For this review, take the finished solid that the model builds, in its own axes (mm). Face numbers are marked on the shaded views. A direction names the side the tool comes from. Round coordinates to 2 decimals unless told otherwise and drop trailing zeros. Order: outer loops, then holes, each group sorted by start corner. A loop starts at its lowest first (then second) coordinate and runs counter-clockwise, first axis right, second up. Notation, with made-up numbers: M 47.5,49.5 L 90.5,49.5 A13 ccw 90.5,69.5 Z; hole C 38.25,78.25 d9. An arc over 180 degrees is marked long. Use a Markdown table: item, result.
from build123d import *

# Parameters (mm, degrees)
BOSS_EXTRUDE1_DEPTH      = 25.8
BOSS_EXTRUDE1_DEPTH_BACK = 25.8
CUT_EXTRUDE2_DEPTH       = 105.5
FILLET3_R                = 2
FILLET2_R                = 5
SKETCH4_R                = 2.3
BOSS_EXTRUDE2_DEPTH      = 9
SKETCH8_W                = 9.403990972
SKETCH8_H                = 11.260041821
SKETCH8_W_2              = 16.148154032
SKETCH8_H_2              = 11.415373045
CUT_EXTRUDE5_DEPTH       = 10
CUT_EXTRUDE6_DEPTH       = 56
CUT_EXTRUDE7_DEPTH       = 56
SKETCH11_W               = 6
SKETCH11_H               = 6
BOSS_EXTRUDE3_DEPTH      = 4
SKETCH12_R               = 1.25
CUT_EXTRUDE8_DEPTH       = 7
SKETCH13_W               = 5
SKETCH13_H               = 2.5
CUT_EXTRUDE9_DEPTH       = 4.5


with BuildPart() as part:
    # Sketch1 → Boss-Extrude1 (new, two sides: drawn at the far end of the back side and taken through both)
    with BuildSketch(Plane(origin=(0, 0, 0), x_dir=(0, 0, -1), z_dir=(1, 0, 0)).offset(-BOSS_EXTRUDE1_DEPTH_BACK)):
        Polygon((-45.5, 0), (-45.5, 21.5), (45.5, 21.5), (45.5, 0), (47.5, 0), (47.5, 23.5), (-47.5, 23.5), (-47.5, 0), align=None)
    extrude(amount=BOSS_EXTRUDE1_DEPTH + BOSS_EXTRUDE1_DEPTH_BACK)

    # Sketch3 → Cut-Extrude2 (cut)
    with BuildSketch(Plane(origin=(0, 0, -47.5), x_dir=(-1, 0, 0), z_dir=(0, 0, -1))):
        Polygon((-25.8, 21.5), (-24.65, 0), (-25.8, 0), align=None)
        Polygon((25.8, 21.5), (24.65, 0), (25.8, 0), align=None)
    extrude(amount=-CUT_EXTRUDE2_DEPTH, mode=Mode.SUBTRACT)

    # Fillet3
    fillet3_edges = [part.edges().sort_by_distance(p)[0] for p in [
        (24.65, 0, -46.5),
        (24.65, 0, 46.5),
        (-24.65, 0, -46.5),
        (-24.65, 0, 46.5),
    ]]
    fillet(fillet3_edges, radius=FILLET3_R)

    # Fillet2
    fillet2_edges = [part.edges().sort_by_distance(p)[0] for p in [
        (0, 21.5, 45.5),
        (0, 23.5, 47.5),
        (0, 23.5, -47.5),
        (0, 21.5, -45.5),
    ]]
    fillet(fillet2_edges, radius=FILLET2_R)

    # Sketch4 → Boss-Extrude2 (add)
    with BuildSketch(Plane.XZ.offset(-21.5)):
        with Locations(Location((-18.5, -26, 0), (0, 0, 270))):
            Circle(SKETCH4_R)
        with Locations(Location((18.5, -26, 0), (0, 0, 270))):
            Circle(SKETCH4_R)
        with Locations(Location((-18.5, 26, 0), (0, 0, 270))):
            Circle(SKETCH4_R)
        with Locations(Location((18.5, 26, 0), (0, 0, 270))):
            Circle(SKETCH4_R)
    extrude(amount=BOSS_EXTRUDE2_DEPTH)

    # Sketch8 → Cut-Extrude5 (cut)
    with BuildSketch(Plane.XY.offset(47.5)):
        with Locations((-10.345619811, 9.988318774)):
            Rectangle(SKETCH8_W, SKETCH8_H)
        with Locations((9.712305605, 7.570757784)):
            Rectangle(SKETCH8_W_2, SKETCH8_H_2)
    extrude(amount=-CUT_EXTRUDE5_DEPTH, mode=Mode.SUBTRACT)

    # Sketch9 → Cut-Extrude6 (cut)
    with BuildSketch(Plane(origin=(25.8, 0, 0), x_dir=(0, 0, -1), z_dir=(1, 0, 0))):
        with BuildLine():
            Line((-22.5, 23.5), (-22.5, 22.498632165))
            Line((-22.5, 22.498632165), (42.604598318, 22.498632165))
            ThreePointArc((42.604598318, 22.498632165), (45.365169565, 21.291201061), (46.5, 18.5))
            Line((46.5, 18.5), (46.5, 1.893175959))
            Line((46.5, 1.893175959), (47.5, 1.893175959))
            Line((47.5, 1.893175959), (47.5, 18.5))
            ThreePointArc((47.5, 18.5), (46.035533906, 22.035533906), (42.5, 23.5))
            Line((42.5, 23.5), (-22.5, 23.5))
        make_face()
    extrude(amount=-CUT_EXTRUDE6_DEPTH, mode=Mode.SUBTRACT)

    # Sketch10 → Cut-Extrude7 (cut)
    with BuildSketch(Plane(origin=(0, 22.498632165, 0), x_dir=(1, 0, 0), z_dir=(0, 1, 0))):
        Polygon((-22.8, -22.5), (-22.8, 21.604598318), (-12.8, 21.604598318), (-12.8, 29.604598318), (-22.8, 29.604598318), (-22.8, 38.604598318), (23.045882962, 38.604598318), (23.045882962, 29.604598318), (13.045882962, 29.604598318), (13.045882962, 21.604598318), (23.045882962, 21.604598318), (23.045882962, -22.5), align=None)
    extrude(amount=-CUT_EXTRUDE7_DEPTH, mode=Mode.SUBTRACT)

    # Sketch11 → Boss-Extrude3 (add)
    with BuildSketch(Plane(origin=(0, 0, -46.5), x_dir=(-1, 0, 0), z_dir=(0, 0, -1))):
        with Locations((-14.195398892, 10.196587979)):
            Rectangle(SKETCH11_W, SKETCH11_H)
        with Locations((14.195398892, 10.196587979)):
            Rectangle(SKETCH11_W, SKETCH11_H)
    extrude(amount=-BOSS_EXTRUDE3_DEPTH)

    # Sketch12 → Cut-Extrude8 (cut)
    with BuildSketch(Plane(origin=(0, 0, -46.5), x_dir=(-1, 0, 0), z_dir=(0, 0, -1))):
        with Locations((14.195398892, 10.196587979)):
            Circle(SKETCH12_R)
        with Locations((-14.195398892, 10.196587979)):
            Circle(SKETCH12_R)
    extrude(amount=-CUT_EXTRUDE8_DEPTH, mode=Mode.SUBTRACT)

    # Sketch13 → Cut-Extrude9 (cut)
    with BuildSketch(Plane(origin=(0, 13.196587979, 0), x_dir=(1, 0, 0), z_dir=(0, 1, 0))):
        with Locations((14.195398892, 44.25)):
            Rectangle(SKETCH13_W, SKETCH13_H)
        with Locations((-14.195398892, 44.25)):
            Rectangle(SKETCH13_W, SKETCH13_H)
    extrude(amount=-CUT_EXTRUDE9_DEPTH, mode=Mode.SUBTRACT)


solid = part.part
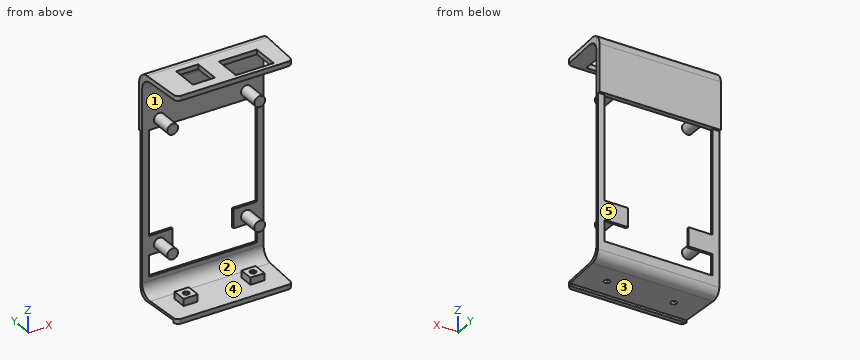
Q1. Draft analysis for pull direction X (two halves, no side actions). For the marked faces 4 and 5, state which applies: pulls with the +X half, pulls with the -X half, needs draft (parallel to the pull), parting line crosses it, or undercut.
Determined:
| item | result |
|---|---|
| face 4 | undercut |
| face 5 | needs draft |
Q2. Add section A-A (x = 0). Write out the cut boundary in (y, z).
Determined:
| item | result |
|---|---|
| outline | M 0,-47.5 L 1.89,-47.5 L 1.89,-46.5 L 18.5,-46.5 A4 ccw 22.5,-42.6 L 22.5,-38.6 L 21.5,-38.6 L 21.5,-40.5 A5 cw 16.5,-45.5 L 0,-45.5 Z; M 0,45.5 L 16.5,45.5 A5 cw 21.5,40.5 L 21.5,22.5 L 23.5,22.5 L 23.5,42.5 A5 ccw 18.5,47.5 L 0,47.5 Z |
Q3. Add section B-B (x = 9.5). Write out the cut boundary in (y, z).
Determined:
| item | result |
|---|---|
| outline | M 0,-47.5 L 1.89,-47.5 L 1.89,-46.5 L 18.5,-46.5 A4 ccw 22.5,-42.6 L 22.5,-38.6 L 21.5,-38.6 L 21.5,-40.5 A5 cw 16.5,-45.5 L 0,-45.5 Z; M 0,45.5 L 1.86,45.5 L 1.86,47.5 L 0,47.5 Z; M 13.28,45.5 L 16.5,45.5 A5 cw 21.5,40.5 L 21.5,22.5 L 23.5,22.5 L 23.5,42.5 A5 ccw 18.5,47.5 L 13.28,47.5 Z |
Q4. Add section D-D (z = 9). Write out the cut boundary in (x, y).
Determined:
| item | result |
|---|---|
| outline | M -25.8,21.5 L -22.8,21.5 L -22.8,22.5 L -25.8,22.5 Z; M 23.05,21.5 L 25.8,21.5 L 25.8,22.5 L 23.05,22.5 Z |
Q5. Wall thickness on line 1 along Z through (x, y) = (21, 8.5); line 2 along Z through (x, y) = (15, 11.5); line 3 along Y through (x, z) = (-6, 29): over which ranges is each line inside the solid? List them lowest first. Write a range as [from, to].
Determined:
| item | result |
|---|---|
| line 1 | z = [-46.5, -45.5], [45.5, 47.5] |
| line 2 | z = [-46.5, -45.5], [-43, -42.5] |
| line 3 | y = [21.5, 23.5] |
Q6. Clearance check with flat-ended pins moving along their axes: pin 1 (8.5 mm diameter, centred on x = 10, y = 10.5, fed in from -Z); pin 2 (1.2 mm diameter, centred on x = -13.5, z = -44.5, fed in from +Y); pin 3 (2.5 mm diameter, centred on y = 9, z = -44.5, fed in from -X). State where each tip first meets the part, or that it passes through.
Determined:
| item | result |
|---|---|
| pin 1 | stops at z = -46.5 |
| pin 2 | stops at y = 22.25 |
| pin 3 | stops at x = -25.17 |
Q7. Machinability: for the marked faces 1, 2 and 3, which of the approach directions +Z, -Z, +X, -X, +Y, -Y give a long, thin tool a straight path to every point of the face, cutting with its end or side? Answer none if there is none.
Determined:
| item | result |
|---|---|
| face 1 | -Y |
| face 2 | +X, -X |
| face 3 | -Z, +X, -X, +Y |
Q8. Add section C-C (z = 26). Write out the cut boundary in (x, y), then the cut area to 3 significant figures.
Determined:
| item | result |
|---|---|
| outline | M -25.8,21.5 L -20.8,21.5 L -20.8,12.5 L -16.2,12.5 L -16.2,21.5 L 16.2,21.5 L 16.2,12.5 L 20.8,12.5 L 20.8,21.5 L 25.8,21.5 L 25.8,23.5 L -25.8,23.5 Z |
| area | 186 mm^2 |
